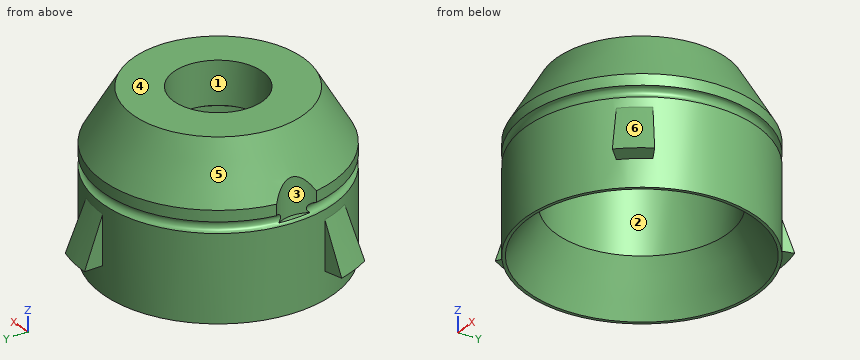
from build123d import *

# Parameters (mm, degrees)
REVOLUTION012_ANGLE = -15
REVOLUTION013_ANGLE = -15
REVOLUTION014_ANGLE = -15
POCKET_DEPTH        = 5
POCKET_DEPTH_BACK   = 3.2
SKETCH139_R         = 5
POCKET046_DEPTH     = 12


with BuildPart() as part:
    # Sketch031 → Revolution010 (revolve)
    with BuildSketch(Plane.YZ):
        with BuildLine():
            Line((14.02, -8), (14.02, -18.5))
            Line((14.02, -18.5), (18.5, -26.259588))
            Line((18.5, -26.259588), (19, -26.259588))
            Line((19, -12.225613), (19, -26.259588))
            ThreePointArc((19, -10.425613), (18.1, -11.325613), (19, -12.225613))
            Line((19, -8.625613), (19, -10.425613))
            Line((19, -8.625613), (14.02, 0))
            Line((14.02, 0), (7.3, 0))
            Line((7.3, 0), (7.3, -7))
            Line((7.3, -7), (9, -7))
            Line((9, -7), (9, -8))
            Line((9, -8), (14.02, -8))
        make_face()
    revolve(axis=Axis((0, 0, 0), (0, 0, 1)))

    # Sketch036 → Revolution012 (revolve)
    with BuildSketch(Plane.YZ):
        Polygon((19, -13.8), (19, -21.8), (22, -21.8), align=None)
    revolve(axis=Axis((0, 0, 0), (0, 0, 1)), revolution_arc=REVOLUTION012_ANGLE)

    # Sketch037 (on DatumPlane) → Revolution013 (revolve)
    with BuildSketch(Plane(origin=(0, 0, 0), x_dir=(-0.866025, -0.5, 0), z_dir=(-0.5, 0.866025, 0))):
        Polygon((19, -13.8), (19, -21.8), (22, -21.8), align=None)
    revolve(axis=Axis((0, 0, 0), (0, 0, 1)), revolution_arc=REVOLUTION013_ANGLE)

    # Sketch038 (on DatumPlane) → Revolution014 (revolve)
    with BuildSketch(Plane(origin=(0, 0, 0), x_dir=(0.866025, -0.5, 0), z_dir=(-0.5, -0.866025, 0))):
        Polygon((19, -13.8), (19, -21.8), (22, -21.8), align=None)
    revolve(axis=Axis((0, 0, 0), (0, 0, 1)), revolution_arc=REVOLUTION014_ANGLE)

    # Sketch062 (on Face24 of Revolution014) → Pocket (cut, two sides)
    with BuildSketch(Plane.YX.offset(7)) as pocket_sk:
        Polygon((7.8, 0), (7.8, 1.5), (13.1, 1.5), (13.1, -1.5), (7.8, -1.5), align=None)
    extrude(amount=POCKET_DEPTH, mode=Mode.SUBTRACT)
    extrude(pocket_sk.sketch, amount=-POCKET_DEPTH_BACK, mode=Mode.SUBTRACT)

    # Sketch139 → Pocket046 (cut)
    with BuildSketch(Plane.XY):
        with Locations((-22.5, 0)):
            Circle(SKETCH139_R)
    extrude(amount=-POCKET046_DEPTH, mode=Mode.SUBTRACT)


with BuildPart() as part_1:
    # Body008 placement: moved
    add(part.part.moved(Location((0, 0, 40))))


solid = part_1.part
Verification items for the finished model (mm, model axes). Face numbers are marked on the shaded views. A direction names the side the tool comes from. Round coordinates to 2 decimals unless told otherwise and drop trailing zeros. Loops run counter-clockwise (first coordinate to the right, second up) from the corner with the lowest first, then second, coordinate; pieces in that order, holes last. Notation, with made-up numbers: (49, -16) - (81, -16) arc R9 ccw to (81, -8) - close; hole circle Ø2 at (69.5, 82). An arc over 180 degrees is marked (long way). Use a Markdown table: item, result. Add a question column.
1. Section check D-D, the plane z = 20.5. Record the boundary of the cut face in (x, y) (1 decimal), plus the area to 3 significant figures.
2. Section check A-A, the plane y = 0. Record the boundary of the cut face in (x, z).
3. Gauge pin test, flat ends, axial feed: pin 1 (2.5 mm diameter, centred on x = -0.5, z = 34, fed in from +Y); pin 2 (2.5 mm diameter, centred on x = 0.5, z = 33, fed in from -Y); pin 3 (12 mm diameter, centred on x = -12, z = 22.5, fed in from -Y). Record the tip position at first contact, or that the pin passes through.
4. Section check C-C, the plane z = 35.5. Record the boundary of the cut face in (x, y), plus the area to 3 significant figures.
5. Access from +Z, -Z, +X, -X, +Y, -Y to the whole of each face (thin tool, end or side, straight path). Record for the marked faces 1 and 2.
6. Thickness scan on probe 1 along X at (y, z) = (0, 27.25); probe 2 along Y at (x, z) = (0, 35); probe 3 along Z at (x, y) = (-8.5, 1.5). Record the ranges inside material, lowest first. Write a range as [from, to].
7. Release check for a two-part mould opening along Y. For the marked faces 3, 4, 5 and 6 record: released by +Y, released by -Y, zero draft, split by the parting line, or undercut.
8. Section check B-B, the plane z = 27. Record the boundary of the cut face in (x, y).
Checks:
| question | item | result |
|---|---|---|
| 1 | outline | (-20.4, -5.5) arc R21.1 ccw to (-18.3, -10.6) - (-16.5, -9.5) arc R19 ccw to (13.4, -13.4) - (14.9, -14.9) arc R21.1 ccw to (18.3, -10.6) - (16.5, -9.5) arc R19 ccw to (4.9, 18.4) - (5.5, 20.4) arc R21.1 ccw to (0, 21.1) - (0, 19) arc R19 ccw to (-18.4, -4.9) - close; hole circle Ø29.2 at (0, 0) |
| 1 | area | 498 mm^2 |
| 2 | outline | (-19, 13.74) - (-18.5, 13.74) - (-14.02, 21.5) - (-14.02, 32) - (-9, 32) - (-9, 33) - (-7.3, 33) - (-7.3, 40) - (-14.02, 40) - (-17.5, 33.97) - (-17.5, 28) - (-18.4, 28) arc R0.9 cw to (-19, 27.77) - close; (7.3, 33) - (9, 33) - (9, 32) - (14.02, 32) - (14.02, 21.5) - (18.5, 13.74) - (19, 13.74) - (19, 27.77) arc R0.9 cw to (19, 29.57) - (19, 31.37) - (14.02, 40) - (7.3, 40) - close |
| 3 | pin 1 | stops at y = 18.2 |
| 3 | pin 2 | stops at y = -18.78 |
| 3 | pin 3 | stops at y = -18.03 |
| 4 | outline | circle Ø33.24 at (0, 0); hole circle Ø14.6 at (0, 0); hole (-1.5, 7.8) - (1.5, 7.8) - (1.5, 13.1) - (-1.5, 13.1) - close |
| 4 | area | 684 mm^2 |
| 5 | face 1 | +Z, -Z |
| 5 | face 2 | -Z |
| 6 | probe 1 | x = [-19, -14.02], [14.02, 19] |
| 6 | probe 2 | y = [-16.91, -7.3], [7.3, 7.8], [13.1, 16.91] |
| 6 | probe 3 | z = [33, 40] |
| 7 | face 3 | undercut |
| 7 | face 4 | zero draft |
| 7 | face 5 | split by the parting line |
| 7 | face 6 | released by -Y |
| 8 | outline | circle Ø38 at (0, 0); hole circle Ø28.04 at (0, 0) |
